The model under review builds one solid part; all positions refer to its coordinate system, in mm. Face numbers are marked on the shaded views. Round coordinates to 2 decimals unless told otherwise and drop trailing zeros. Order: outer loops, then holes, each group sorted by start corner. A loop starts at its lowest first (then second) coordinate and runs counter-clockwise, first axis right, second up. Notation, with made-up numbers: M 25.25,77 L 78.25,77 A6 ccw 78.25,81 Z; hole C 69.5,-29.75 d1. An arc over 180 degrees is marked long. Answer as a JSON object with one key per item and string values. Group by question number.
1) Consider section C-C, the plane x = -4. Write out the cut boundary in (y, z).
2) Insertion check: pin 1 Ø6 at (x, y) = (32.5, -32) entering from +Z; pin 2 Ø10 at (x, z) = (27.5, 13) entering from +Y; pin 3 Ø7.5 at (x, y) = (56.89, 28.58) entering from +Z; pin 4 Ø17.5 at (x, y) = (56.89, -28.58) entering from -Z. Each pin has a flat end and moves straight along its axis. Give the tip position at first contact, or say it passes through.
3) To check wall thickness, follow line 1 (X direction, y = 0.5, z = 34); line 2 (Z direction, x = 23.5, y = -12.5); line 3 (Y direction, x = -7.5, z = 32.5). State the ranges of each line that lie inside material, in increasing order.
4) Consider section D-D, the plane z = 21.5. Write out the cut boundary in (x, y) (1 decimal), then the cut area to 3 significant figures.
5) Consider section B-B, the plane y = -33.5. Write out the cut boundary in (x, z).
6) The part is to be moulded in two halves that separate along Y. For the marked faces 1, 2 and 3, say which applies: +Y half, -Y half, draft (parallel to the pull), parting line (faces both ways), or undercut.
7) Consider section A-A, the plane z = 3.5. Write out the cut boundary in (x, y) (1 decimal), then the cut area to 3 significant figures.
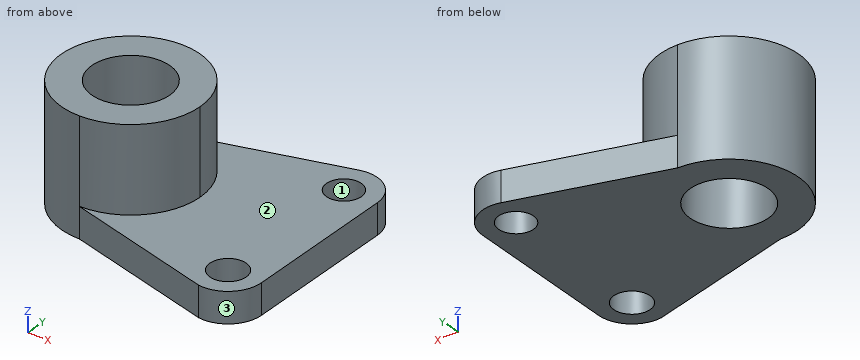
```python
from build123d import *

# Parameters (mm, degrees)
F0_R     = 14.2875
F1_DEPTH = 42.2148
F0_R_2   = 6.669194
F0_R_3   = 6.405374
F2_DEPTH = 11.176


with BuildPart() as f1:
    # F0 (on Top) → F1 (new body)
    with BuildSketch(Plane.XY):
        with BuildLine():
            ThreePointArc((0, -25.4), (17.960512, -17.960512), (25.4, 0))
            ThreePointArc((25.4, 0), (17.960512, 17.960512), (0, 25.4))
            ThreePointArc((0, 25.4), (-25.4, 0), (0, -25.4))
        make_face()
        Circle(F0_R, mode=Mode.SUBTRACT)
    extrude(amount=F1_DEPTH)

    # F0 (on Top) → F2 (join)
    with BuildSketch(Plane.XY):
        with BuildLine():
            ThreePointArc((0, 25.4), (17.960512, 17.960512), (25.4, 0))
            ThreePointArc((25.4, 0), (17.960512, -17.960512), (0, -25.4))
            Line((0, -25.4), (55.144853, -40.682886))
            ThreePointArc((55.144853, -40.682886), (64.902158, -37.823193), (69.127533, -28.575))
            Line((69.127533, -28.575), (69.127533, 28.575))
            ThreePointArc((69.127533, 28.575), (64.304451, 38.308701), (53.638201, 40.367384))
            Line((53.638201, 40.367384), (0, 25.4))
        make_face()
        with Locations((56.893961, -28.575)):
            Circle(F0_R_2, mode=Mode.SUBTRACT)
        with Locations((56.893961, 28.575)):
            Circle(F0_R_3, mode=Mode.SUBTRACT)
    extrude(amount=F2_DEPTH)


solid = f1.part
```
Results list:
{
 "1": {"outline": "M -25.08,0 L -13.72,0 L -13.72,42.21 L -25.08,42.21 Z; M 13.72,0 L 25.08,0 L 25.08,42.21 L 13.72,42.21 Z"},
 "2": {"pin 1": "z = 11.18", "pin 2": "y = 34.37", "pin 3": "through", "pin 4": "z = 0"},
 "3": {"line 1": "-25.4 to -14.28, 14.28 to 25.4", "line 2": "0 to 11.18", "line 3": "-24.27 to -12.16, 12.16 to 24.27"},
 "4": {"outline": "M 0,-25.4 A25.4 ccw 25.4,0 A25.4 ccw long Z; hole C 0,0 d28.6", "area": "1,390 mm^2"},
 "5": {"outline": "M 29.23,0 L 52.4,0 L 52.4,11.18 L 29.23,11.18 Z; M 61.39,0 L 68.09,0 L 68.09,11.18 L 61.39,11.18 Z"},
 "6": {"face 1": "undercut", "face 2": "draft", "face 3": "-Y half"},
 "7": {"outline": "M 0,-25.4 L 55.1,-40.7 A12.2 ccw 69.1,-28.6 L 69.1,28.6 A12.2 ccw 53.6,40.4 L 0,25.4 A25.4 ccw Z; hole C 0,0 d28.6; hole C 56.9,-28.6 d13.3; hole C 56.9,28.6 d12.8", "area": "4,830 mm^2"}
}
